For this review, take the finished solid that the model builds, in its own axes (mm). A direction names the side the tool comes from. Round coordinates to 2 decimals unless told otherwise and drop trailing zeros. Write each loop counter-clockwise with the first axis right and the second up, starting at its lowest first coordinate (ties: lowest second). Pieces come first, ordered by that corner, then holes. Notation, with made-up numbers: (83.25, 51) -> (117.25, 51) arc R33 ccw to (117.25, 84) -> close; hole circle Ø1 at (-29.5, 43.5). An arc over 180 degrees is marked (long way). Answer in a Markdown table with one row per item.
from build123d import *

# Parameters (mm, degrees)
F0_W           = 105
F0_H           = 55
F1_DEPTH       = 25
F2_D           = 10
F2_DEPTH       = 15
F2_TIP         = 3.0043030951
F3_D           = 5
F3_DEPTH       = 20
F3_TIP         = 1.5021515476
F4_W           = 15
F4_H           = 55
F4_W_2         = 17.9679095745
F4_H_2         = 55.3074888885
F5_DEPTH       = 60
F6_R           = 16.1752308679
F9_D           = 20
F9_DEPTH       = 50
F9_TIP         = 6.0086061903
F9_ON_F8_D     = 20
F9_ON_F8_DEPTH = 50
F9_ON_F8_TIP   = 6.0086061903
F10_W          = 22.9570271527
F10_H          = 60
F10_R          = 10
F11_DEPTH      = 1
F13_DEPTH      = 1


with BuildPart() as f1:
    # F0 (on Top) → F1 (new body)
    with BuildSketch(Plane.XY):
        Rectangle(F0_W, F0_H)
    extrude(amount=F1_DEPTH)

    # F2
    with Locations(Plane(origin=(0, 0, 0), x_dir=(1, 0, 0), z_dir=(0, 0, -1))):
        with Locations((-9.5454547554, -13.6163104326), (-9.5454547554, 16.7045462877), (10.4545452446, -13.6163104326), (10.4545452446, 17.2660425305)):
            Hole(F2_D / 2, depth=F2_DEPTH)
            with Locations((0, 0, -(F2_DEPTH + F2_TIP / 2))):  # 118° drill point
                Cone(0, F2_D / 2, F2_TIP, mode=Mode.SUBTRACT)

    # F3
    with Locations(Plane(origin=(0, 0, 0), x_dir=(1, 0, 0), z_dir=(0, 0, -1))):
        with Locations((-9.5454547554, 16.7045462877), (10.4545452446, 17.2660425305)):
            Hole(F3_D / 2, depth=F3_DEPTH)
            with Locations((0, 0, -(F3_DEPTH + F3_TIP / 2))):  # 118° drill point
                Cone(0, F3_D / 2, F3_TIP, mode=Mode.SUBTRACT)

    # F4 (on face) → F5 (join)
    with BuildSketch(Plane.XY):
        with Locations((-45.2807511389, -0.1537444443)):
            Rectangle(F4_W, F4_H)
        with Locations((43.7967926264, 0)):
            Rectangle(F4_W_2, F4_H_2)
    extrude(amount=-F5_DEPTH)

    # F6
    f6_edges = [f1.edges().sort_by_distance(p)[0] for p in [
        (-45.280751, 27.346256, -60),
        (-45.280751, -27.653744, -60),
        (43.796793, -27.653744, -60),
        (43.796793, 27.653744, -60),
    ]]
    fillet(f6_edges, radius=F6_R)

    # F9 (one way)
    with BuildSketch(Plane(origin=(34.8128378391, 0, 0), x_dir=(0, -1, 0), z_dir=(-1, 0, 0))):
        with Locations((0, -40.2935221791)):
            Circle(F9_D / 2)
    extrude(amount=-F9_DEPTH, mode=Mode.SUBTRACT)
    with Locations(Plane(origin=(34.8128378391, 0, 0), x_dir=(0, -1, 0), z_dir=(-1, 0, 0))):
        with Locations((0, -40.2935221791)):
            with Locations((0, 0, -(F9_DEPTH + F9_TIP / 2))):  # 118° drill point
                Cone(0, F9_D / 2, F9_TIP, mode=Mode.SUBTRACT)

    # F9 on F8 (one way)
    with BuildSketch(Plane.YZ.offset(-37.7807511389)):
        with Locations((0, -40.3322502971)):
            Circle(F9_ON_F8_D / 2)
    extrude(amount=-F9_ON_F8_DEPTH, mode=Mode.SUBTRACT)
    with Locations(Plane.YZ.offset(-37.7807511389)):
        with Locations((0, -40.3322502971)):
            with Locations((0, 0, -(F9_ON_F8_DEPTH + F9_ON_F8_TIP / 2))):  # 118° drill point
                Cone(0, F9_ON_F8_D / 2, F9_ON_F8_TIP, mode=Mode.SUBTRACT)

    # F10 (on face) → F11 (cut)
    with BuildSketch(Plane.YZ.offset(52.7807474136)):
        with Locations((0, -30)):
            Rectangle(F10_W, F10_H)
        with Locations((0, -40.2935221791)):
            Circle(F10_R, mode=Mode.SUBTRACT)
    extrude(amount=-F11_DEPTH, mode=Mode.SUBTRACT)

    # F12 (on face) → F13 (cut)
    with BuildSketch(Plane(origin=(-52.5, 0, 0), x_dir=(0, -1, 0), z_dir=(-1, 0, 0))):
        with BuildLine():
            Line((-8.1417122856, 13.3355623111), (8.7032085285, 13.8970594853))
            ThreePointArc((8.7032085285, 13.8970594853), (0.0070411683, 21.8275222154), (-8.1417122856, 13.3355623111))
        make_face()
        Polygon((15, -58.8169405147), (8.7032085285, 13.8970594853), (-8.1417122856, 13.3355623111), (-15, -59.3783445656), align=None)
    extrude(amount=-F13_DEPTH, mode=Mode.SUBTRACT)


solid = f1.part
1) Consider section C-C on x = -45.5. State the section outline as (y, z) points, then the cut area to 3 significant figures.
Solved:
| item | result |
|---|---|
| outline | (-27.65, -43.82) arc R16.18 ccw to (-11.48, -60) -> (11.17, -60) arc R16.18 ccw to (27.35, -43.82) -> (27.35, 0) -> (27.5, 0) -> (27.5, 25) -> (-27.5, 25) -> (-27.5, 0) -> (-27.65, 0) -> close; hole circle Ø20 at (0, -40.33) |
| area | 4,250 mm² |
2) Consider section A-A on z = -16.5. State the section outline as (x, y) points, then the cut area to 3 significant figures.
Solved:
| item | result |
|---|---|
| outline | (-52.78, -27.65) -> (-37.78, -27.65) -> (-37.78, 27.35) -> (-52.78, 27.35) -> close; (34.81, -27.65) -> (52.78, -27.65) -> (52.78, -11.48) -> (51.78, -11.48) -> (51.78, 11.48) -> (52.78, 11.48) -> (52.78, 27.65) -> (34.81, 27.65) -> close; hole (-52.5, -11.34) -> (-51.5, -11.34) -> (-51.5, 10.96) -> (-52.5, 10.96) -> close |
| area | 1,770 mm² |
3) Clearance check with flat-ended pins moving along their axes: pin 1 Ø6 at (x, y) = (4.5, -21) entering from -Z; pin 2 Ø2 at (y, z) = (-18.5, 8) entering from -X; pin 3 Ø2 at (x, y) = (-9.5, -19.5) entering from -Z. State where each tip first meets the part, or that it passes through.
Solved:
| item | result |
|---|---|
| pin 1 | z = 0 |
| pin 2 | x = -52.5 |
| pin 3 | z = 15.72 |
4) Consider section D-D on y = 0. State the section outline as (x, z) points, then the cut area to 3 significant figures.
Solved:
| item | result |
|---|---|
| outline | (-52.78, -60) -> (-37.78, -60) -> (-37.78, -50.33) -> (-51.5, -50.33) -> (-51.5, -59.1) -> (-52.5, -59.1) -> (-52.5, -50.33) -> (-52.78, -50.33) -> close; (-52.78, -30.33) -> (-52.5, -30.33) -> (-52.5, 0) -> (-52.78, 0) -> close; (-52.5, 21.83) -> (-51.5, 21.83) -> (-51.5, -30.33) -> (-37.78, -30.33) -> (-37.78, 0) -> (34.81, 0) -> (34.81, -30.29) -> (51.78, -30.29) -> (51.78, 0) -> (52.5, 0) -> (52.5, 25) -> (-52.5, 25) -> close; (34.81, -60) -> (51.78, -60) -> (51.78, -50.29) -> (34.81, -50.29) -> close |
| area | 3,840 mm² |
5) For faces 1 (the flat face through (-51.5, 0, -18)), 2 (the cylindrical face through (-8.89, -21.66, 7.6)), 3 (the flat face through (-1, -27.5, 12)), list the 3-axis set-ups (+Z, -Z, +X, -X, +Y, -Y) from which the entire face can be reached by the end or side of a thin tool; tool diameter is ignored.
Solved:
| item | result |
|---|---|
| face 1 | none |
| face 2 | -Z |
| face 3 | +Z, +X, -X, -Y |
6) For line 1 (X direction, y = -4.5, z = -19); line 2 (X direction, y = -18.5, z = -40); line 3 (Z direction, x = 42, y = 0), list the stretches that pass through material, from the lowest coordinate up. Write a range as [from, to].
Solved:
| item | result |
|---|---|
| line 1 | [-52.78, -52.5], [-51.5, -37.78], [34.81, 51.78] |
| line 2 | [-52.78, -37.78], [34.81, 52.78] |
| line 3 | [-60, -50.29], [-30.29, 25] |
7) Mouldability with a two-part tool opening along X and no side actions: class faces 4 (the cylindrical face through (43.92, -23.04, -55.14)), 5 (the flat face through (-37.781, -1, -30)) as pulls with the +X half, pulls with the -X half, needs draft (parallel to the pull), parting line crosses it, or undercut.
Solved:
| item | result |
|---|---|
| face 4 | needs draft |
| face 5 | undercut |
8) Consider section B-B on z = -37. State the section outline as (x, y) points, then the cut area to 3 significant figures.
Solved:
| item | result |
|---|---|
| outline | (-52.78, -27.65) -> (-37.78, -27.65) -> (-37.78, -9.43) -> (-51.5, -9.43) -> (-51.5, -13.11) -> (-52.5, -13.11) -> (-52.5, -9.43) -> (-52.78, -9.43) -> close; (-52.78, 9.43) -> (-52.5, 9.43) -> (-52.5, 12.89) -> (-51.5, 12.89) -> (-51.5, 9.43) -> (-37.78, 9.43) -> (-37.78, 27.35) -> (-52.78, 27.35) -> close; (34.81, -27.65) -> (52.78, -27.65) -> (52.78, -11.48) -> (51.78, -11.48) -> (51.78, -9.44) -> (34.81, -9.44) -> close; (34.81, 9.44) -> (51.78, 9.44) -> (51.78, 11.48) -> (52.78, 11.48) -> (52.78, 27.65) -> (34.81, 27.65) -> close |
| area | 1,190 mm² |
